from build123d import *

# Parameters (mm, degrees)
SKETCH_1_R      = 26
SKETCH_1_R_2    = 1.5
EXTRUDE_1_DEPTH = 3


with BuildPart() as part:
    # Эскиз1 → Бобышка-Вытянуть1 (new body)
    with BuildSketch(Plane(origin=(0, 0, 0), x_dir=(1, 0, 0), z_dir=(0, 1, 0))):
        with Locations(Location((-42.952158514, 15.778810529, 0), (0, 0, 270))):
            Circle(SKETCH_1_R)
        with Locations(Location((-58.452158514, 31.278810529, 0), (0, 0, 270))):
            Circle(SKETCH_1_R_2, mode=Mode.SUBTRACT)
        with Locations(Location((-58.452158514, 0.278810529, 0), (0, 0, 270))):
            Circle(SKETCH_1_R_2, mode=Mode.SUBTRACT)
        with Locations(Location((-27.452158514, 31.278810529, 0), (0, 0, 270))):
            Circle(SKETCH_1_R_2, mode=Mode.SUBTRACT)
        with Locations(Location((-27.452158514, 0.278810529, 0), (0, 0, 270))):
            Circle(SKETCH_1_R_2, mode=Mode.SUBTRACT)
        with BuildLine():
            Line((-46.074657514, 18.278810529), (-39.829659515, 18.278810529))
            ThreePointArc((-39.829659515, 18.278810529), (-42.952158514, 11.778810529), (-46.074657514, 18.278810529))
        make_face(mode=Mode.SUBTRACT)
    extrude(amount=EXTRUDE_1_DEPTH)


solid = part.part
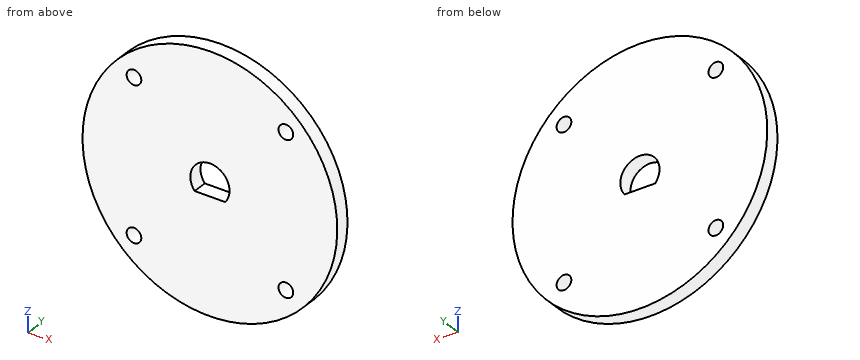
Check sheet for the modelled part. Datum: model origin and axes. Units: mm. Coordinates: 2 decimals unless noted, no trailing zeros. Write each loop counter-clockwise with the first axis right and the second up, starting at its lowest first coordinate (ties: lowest second). Pieces come first, ordered by that corner, then holes.
Item 1: Cross-section at A-A on z = -1. Record the boundary of the cut face in (x, y), then the cut area to 3 significant figures.
Numbers:
outline: (-64.34, 0) - (-59.77, 0) - (-59.77, 3) - (-64.34, 3) - close; (-57.14, 0) - (-28.77, 0) - (-28.77, 3) - (-57.14, 3) - close; (-26.14, 0) - (-21.56, 0) - (-21.56, 3) - (-26.14, 3) - close
area: 113 mm2
Item 2: Cross-section at B-B on x = -45. Record the boundary of the cut face in (y, z), then the cut area to 3 significant figures.
Numbers:
outline: (0, -41.7) - (3, -41.7) - (3, -18.28) - (0, -18.28) - close; (0, -12.34) - (3, -12.34) - (3, 10.14) - (0, 10.14) - close
area: 138 mm2
Item 3: Cross-section at C-C on y = 0.65. Record the boundary of the cut face in (x, z), then the cut area to 3 significant figures.
Numbers:
outline: circle Ø52 at (-42.95, -15.78); hole circle Ø3 at (-58.45, -31.28); hole circle Ø3 at (-58.45, -0.28); hole (-46.07, -18.28) - (-39.83, -18.28) arc R4 ccw (long way) to start; hole circle Ø3 at (-27.45, -31.28); hole circle Ø3 at (-27.45, -0.28)
area: 2,050 mm2
Item 4: Cross-section at D-D on x = -51.5. Record the boundary of the cut face in (y, z), then the cut area to 3 significant figures.
Numbers:
outline: (0, -40.33) - (3, -40.33) - (3, 8.78) - (0, 8.78) - close
area: 147 mm2
Item 5: Scan lines: probe 1 along X at (y, z) = (1, -30); probe 2 along X at (y, z) = (0.8, 1); probe 3 along Z at (x, y) = (-29, 1.2). Record each from-to range of solid material in increasing order.
Numbers:
probe 1: x = -64.72 to -59.24, -57.67 to -28.24, -26.67 to -21.19
probe 2: x = -62.81 to -59.24, -57.67 to -28.24, -26.67 to -23.09
probe 3: z = -37.72 to 6.16
Item 6: Depth check by flat-ended pin: pin 1 Ø1.5 at (x, y) = (-41, 2.5) entering from +Z; pin 2 Ø4 at (x, z) = (-58.45, -31.28) entering from -Y; pin 3 Ø1 at (x, y) = (-24.5, 1.5) entering from -Z; pin 4 Ø1.5 at (x, y) = (-49, 1.5) entering from +Z. Enter the tip coordinate at first touch or a pass-through.
Numbers:
pin 1: stops at z = 10.19
pin 2: stops at y = 0
pin 3: stops at z = -34.59
pin 4: stops at z = 9.68
